Solid Edge part; units mm, degrees
sketch "Sketch1" plane through (0, 0, 0) normal (0, 0, 1) x (1, 0, 0)
  line L0 (-75.7, -40) -> (75.7, -40)
  line L1 (75.7, -40) -> (75.7, 40)
  line L2 (75.7, 40) -> (-75.7, 40)
  line L3 (-75.7, 40) -> (-75.7, -40)
extrude "Protrusion1" add sketch "Sketch1" along normal blind 4
sketch "Sketch2" plane through (0, 0, 0) normal (0, 0, -1) x (1, 0, 0)
  line L0 (-75.7, -40) -> (75.7, -40)
  line L1 (75.7, -40) -> (75.7, 40)
  line L2 (75.7, 40) -> (-75.7, 40)
  line L3 (-75.7, 40) -> (-75.7, -40)
  line L4 (71.7, 36) -> (-71.7, 36)
  line L5 (-71.7, 36) -> (-71.7, -36)
  line L6 (-71.7, -36) -> (71.7, -36)
  line L7 (71.7, -36) -> (71.7, 36)
extrude "Protrusion2" add sketch "Sketch2" along normal blind 16
sketch "Sketch3" plane through (-75.7, 0, -6) normal (-1, 0, 0) x (0, -1, 0)
  line L0 (-3, -10) -> (7.5, -10)
  line L1 (7.5, -10) -> (7.5, -5)
  line L2 (7.5, -5) -> (4.5, -5)
  line L3 (4.5, -5) -> (4.5, 2)
  line L4 (4.5, 2) -> (0, 2)
  line L5 (0, 2) -> (0, -5)
  line L6 (0, -5) -> (-3, -5)
  line L7 (-3, -5) -> (-3, -10)
  line L8 (18.5, -10) -> (29, -10)
  line L9 (29, -10) -> (29, -5)
  line L10 (29, -5) -> (26, -5)
  line L11 (26, -5) -> (26, 2)
  line L12 (26, 2) -> (21.5, 2)
  line L13 (21.5, 2) -> (21.5, -5)
  line L14 (21.5, -5) -> (18.5, -5)
  line L15 (18.5, -5) -> (18.5, -10)
  line L16 (-29, -10) -> (-12.5, -10)
  line L17 (-12.5, -10) -> (-12.5, 1.5)
  line L18 (-12.5, 1.5) -> (-29, 1.5)
  line L19 (-29, 1.5) -> (-29, -10)
  dimension "D1" = 12.5
  dimension "D2" = 21.5
  dimension "D3" = 18.5
  dimension "D4" = 12.5
  dimension "D5" = 4.5
  dimension "D6" = 26
  dimension "D7" = 4.5
  dimension "D8" = 26
  dimension "D9" = 12.5
  dimension "D10" = 7.5
extrude "Cutout1" cut sketch "Sketch3" against normal up to next
sketch "Sketch4" plane through (71.7, 0, -8) normal (-1, 0, 0) x (0, -1, 0)
  circle A0 centre (-10.8, -8) radius 3.5
  dimension "D1" = 10.8
extrude "Cutout2" cut sketch "Sketch4" against normal up to next
sketch "Sketch5" plane through (0, 24.15, -16) normal (0, 0, -1) x (0, -1, 0)
  line L0 (-11.85, 71.7) -> (60.15, 71.7)
  line L1 (60.15, 71.7) -> (60.15, -71.7)
  line L2 (60.15, -71.7) -> (-11.85, -71.7)
  line L3 (-11.85, -71.7) -> (-11.85, 71.7)
  line L4 (-13.85, 73.7) -> (62.15, 73.7)
  line L5 (62.15, 73.7) -> (62.15, -73.7)
  line L6 (62.15, -73.7) -> (-13.85, -73.7)
  line L7 (-13.85, -73.7) -> (-13.85, 73.7)
extrude "ExtrudedCutout_3" cut sketch "Sketch5" against normal blind 2
fillet "Round_1" radius 3 8 edges at (75.7, -40, -6) (75.7, 0, 4) (0, -40, 4) (-75.7, 0, 4) (0, 40, 4) (-75.7, 40, -6) (-75.7, -40, -6) (75.7, 40, -6)
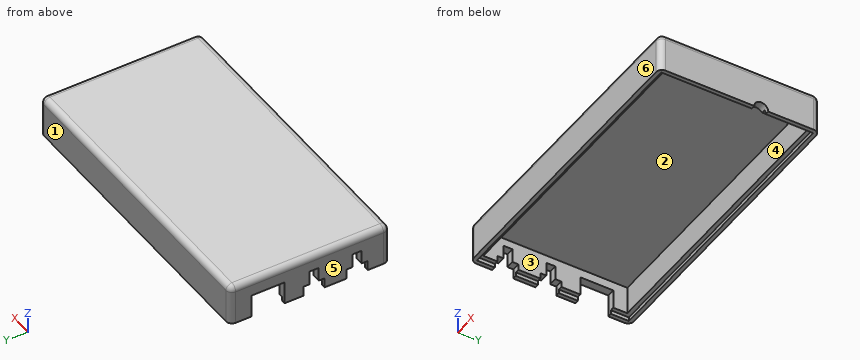
Build history of the part. All positions in model axes, mm. Face numbers are marked on the shaded views. A direction names the side the tool comes from. Round coordinates to 2 decimals unless told otherwise and drop trailing zeros. Write each loop counter-clockwise with the first axis right and the second up, starting at its lowest first coordinate (ties: lowest second). Pieces come first, ordered by that corner, then holes. Notation, with made-up numbers: M 63.25,-32.5 L 81.25,-32.5 A31 ccw 81.25,3.5 Z; hole C 71.25,-18 d4. An arc over 180 degrees is marked long. Use CSV: the item, a comma, the result in double quotes.
1. Saw through at C-C (y = 10.8). Give the cut face in (x, z).
Reply:
outline,"M -75.7,-16 L -73.7,-16 L -73.7,-14 L -71.7,-14 L -71.7,0 L 71.7,0 L 71.7,-12.5 L 75.7,-12.5 L 75.7,1 A3 ccw 72.7,4 L -72.7,4 A3 ccw -75.7,1 Z"
2. Saw through at A-A (y = 32.5). Give the cut face in (x, z).
Reply:
outline,"M -75.7,-16 L -73.7,-16 L -73.7,-14 L -71.7,-14 L -71.7,0 L 71.7,0 L 71.7,-14 L 73.7,-14 L 73.7,-16 L 75.7,-16 L 75.7,1 A3 ccw 72.7,4 L -72.7,4 A3 ccw -75.7,1 Z"
3. Tool access for the marked faces 1 and 2: list every direction of +Z, -Z, +X, -X, +Y, -Y with a clear straight run to the whole face (end or side of a thin tool).
Reply:
face 1,"+Z, -Z, +X, -X, +Y"
face 2,"-Z"
4. Flat gauge pins, fed straight in: pin 1 (1.2 mm diameter, centred on x = -74.5, z = -8.5, fed in from -Y); pin 2 (5 mm diameter, centred on x = 31, y = 13, fed in from -Z); pin 3 (1.2 mm diameter, centred on x = -74, z = -13.5, fed in from -Y). Where does each tip first touch, or does it go through?
Reply:
pin 1,"stops at y = -39.75"
pin 2,"stops at z = 0"
pin 3,"stops at y = -39.92"
5. Wall check: probe 1 along Y at (x, z) = (-64, -0.25); probe 2 along X at (y, z) = (1, -8); probe 3 along X at (y, z) = (-15, -14.5). Give the ranges that are in metal, low to high. Write a range as from..to.
Reply:
probe 1,"y = -40..-36, 36..40"
probe 2,"x = -75.7..-71.7, 71.7..75.7"
probe 3,"x = -75.7..-73.7, 73.7..75.7"
6. Saw through at B-B (x = -24). Give the cut face in (y, z), plus the area to 3 significant figures.
Reply:
outline,"M -40,-16 L -38,-16 L -38,-14 L -36,-14 L -36,0 L 36,0 L 36,-14 L 38,-14 L 38,-16 L 40,-16 L 40,1 A3 ccw 37,4 L -37,4 A3 ccw -40,1 Z"
area,"436 mm²"
7. Two-plate mould, pull along X, no slides. Class the marked faces 3, 4, 5 and 6: +X half, -X half, draft (parallel to the pull), parting line (faces both ways), or undercut.
Reply:
face 3,"undercut"
face 4,"undercut"
face 5,"-X half"
face 6,"draft"
